from build123d import *

# Parameters (mm, degrees)
SHELL1_OUTLINE_R        = 79.375
SHELL1_DEPTH            = 31.75
CUT_EXTRUDE2_REACH      = 143.848
CUT_EXTRUDE2_END_RADIUS = 92.075


# Read off the part's stored shape, not the designer's step: Shell1
with BuildPart() as part:
    # Sketch1 → Revolve1 (revolve)
    with BuildSketch(Plane.XY, mode=Mode.PRIVATE) as revolve1_sk:
        Polygon((0, 0), (92.075, 0), (92.075, 19.05), (95.25, 19.05), (95.25, 44.45), (0, 44.45), align=None)
    revolve(revolve1_sk.sketch.rotate(Axis((0, 0, 0), (0, 1, 0)), 90), axis=Axis((0, 0, 0), (0, 1, 0)))

    # Shell1 outline → Shell1 (cut)
    with BuildSketch(Plane(origin=(0, 0, 0), x_dir=(1, 0, 0), z_dir=(0, 1, 0))):
        Circle(SHELL1_OUTLINE_R)
    extrude(amount=SHELL1_DEPTH, mode=Mode.SUBTRACT)

    # Cut-Extrude2: up to this cylinder (the profile starts inside it)
    cut_extrude2_end = Plane(origin=(0, 0, 0), z_dir=(0, -1, 0)) * Cylinder(CUT_EXTRUDE2_END_RADIUS, 472.846, mode=Mode.PRIVATE)
    # Sketch2 → Cut-Extrude2 (cut, up to the surface)
    with BuildSketch(Plane(origin=(0, 0, 0), x_dir=(0, 0, -1), z_dir=(1, 0, 0)), mode=Mode.PRIVATE) as cut_extrude2_sk1:
        with BuildLine():
            Line((-48.830201285, -11.43), (-48.830201285, 11.43))
            ThreePointArc((-48.830201285, 11.43), (-42.480201285, 17.78), (-36.130201285, 11.43))
            Line((-36.130201285, 11.43), (-36.130201285, -11.43))
            ThreePointArc((-36.130201285, -11.43), (-42.480201285, -17.78), (-48.830201285, -11.43))
        make_face()
    cut_extrude2_tool1 = extrude(cut_extrude2_sk1.sketch, amount=CUT_EXTRUDE2_REACH, mode=Mode.PRIVATE) & cut_extrude2_end
    add(cut_extrude2_tool1.solids().sort_by_distance((0, 0, 42.480201))[0], mode=Mode.SUBTRACT)
    # Sketch2 → Cut-Extrude2 (cut, up to the surface)
    with BuildSketch(Plane(origin=(0, 0, 0), x_dir=(0, 0, -1), z_dir=(1, 0, 0)), mode=Mode.PRIVATE) as cut_extrude2_sk2:
        with BuildLine():
            Line((15.101598715, -11.43), (15.101598715, 11.43))
            ThreePointArc((15.101598715, 11.43), (21.451598715, 17.78), (27.801598715, 11.43))
            Line((27.801598715, 11.43), (27.801598715, -11.43))
            ThreePointArc((27.801598715, -11.43), (21.451598715, -17.78), (15.101598715, -11.43))
        make_face()
    cut_extrude2_tool2 = extrude(cut_extrude2_sk2.sketch, amount=CUT_EXTRUDE2_REACH, mode=Mode.PRIVATE) & cut_extrude2_end
    add(cut_extrude2_tool2.solids().sort_by_distance((0, 0, -21.451599))[0], mode=Mode.SUBTRACT)


solid = part.part
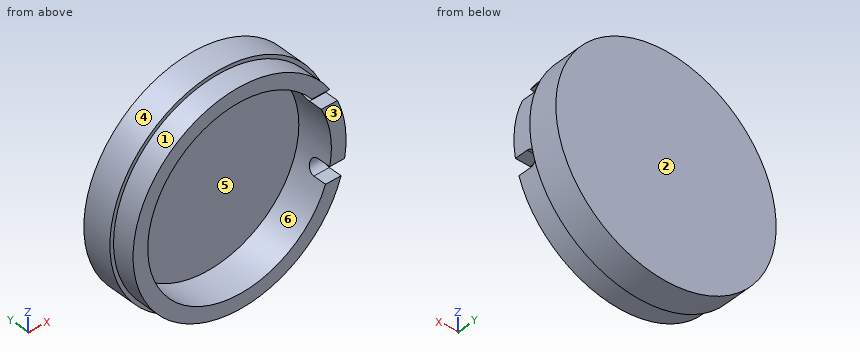
Can you work these out from the model? Positions are in its coordinate system, mm. Face numbers are marked on the shaded views. A direction names the side the tool comes from. Round coordinates to 2 decimals unless told otherwise and drop trailing zeros. Write each loop counter-clockwise with the first axis right and the second up, starting at its lowest first coordinate (ties: lowest second). Pieces come first, ordered by that corner, then holes. Notation, with made-up numbers: (-24, -15.75) -> (4, -15.75) arc R9 ccw to (4, -8.75) -> close; hole circle Ø9 at (40, 32.5). An arc over 180 degrees is marked (long way). Use one line per item in the form item = value. Start each with the question number.
Q1. Imagine slicing it at B-B (z = 0). Please give me the cut outline in (x, y) (3 decimals).
Q2. If I drill on probe 1 along X at (y, z) = (15, 0) (3 decimals); probe 2 along X at (y, z) = (22, 0) (3 decimals); probe 3 along Y at (x, z) = (14, -31.5), over which ranges is the centre line in solid material (lowest first)? Write a range as [from, to].
Q3. We'd pull the mould along Z, two halves only. Please class the marked faces 3, 4, 5 and 6: +Z half, -Z half, draft (parallel to the pull), parting line (faces both ways), or undercut.
Q4. Imagine slicing it at C-C (x = 0). Please give me the cut outline in (y, z) (3 decimals), then the cut area to 3 significant figures.
Q5. I'm going to push flat-ended pins straight in: P1, Ø1.5, axis at x = -27.5, y = 21, coming from the -Z side; P2, Ø3.5, axis at x = 80.5, y = 8.5, coming from the +Z side; P3, Ø1.5, axis at y = 38.5, z = 64, coming from the -X side. Where does each tip first touch, or does it pass through?
Q6. Imagine slicing it at D-D (y = 28). Please give me the cut outline in (x, z) (3 decimals).
Q7. Which directions (+Z, -Z, +X, -X, +Y, -Y) give clear straight access to the entire face, cutting with the end or side of a thin tool? Please do the marked faces 1 and 2.
Q8. Imagine slicing it at A-A (y = 4). Please give me the cut outline in (x, z) (3 decimals).
Worked out:
q1.outline = (-95.25, 19.05) -> (-92.075, 19.05) -> (-92.075, 0) -> (-79.375, 0) -> (-79.375, 31.75) -> (79.375, 31.75) -> (79.375, 0) -> (92.075, 0) -> (92.075, 19.05) -> (95.25, 19.05) -> (95.25, 44.45) -> (-95.25, 44.45) -> close
q2.probe_1 = [-92.075, -79.375], [79.375, 92.075]
q2.probe_2 = [-95.25, -79.375], [79.375, 95.25]
q2.probe_3 = [31.75, 44.45]
q3.face_3 = draft
q3.face_4 = parting line
q3.face_5 = undercut
q3.face_6 = undercut
q4.outline = (0, -92.075) -> (19.05, -92.075) -> (19.05, -95.25) -> (44.45, -95.25) -> (44.45, 95.25) -> (19.05, 95.25) -> (19.05, 92.075) -> (0, 92.075) -> (0, 79.375) -> (31.75, 79.375) -> (31.75, -79.375) -> (0, -79.375) -> close
q4.area = 3,310 mm^2
q5.P1 = -91.42
q5.P2 = 36.13
q5.P3 = -71.22
q6.outline = circle Ø190.5 at (0, 0); hole circle Ø158.75 at (0, 0)
q7.face_1 = -Y
q7.face_2 = +Z, -Z, +X, -X, +Y
q8.outline = (62.578, 48.83) -> (78.06, 48.83) arc R92.075 ccw (long way) to (87.777, -27.802) -> (74.347, -27.802) arc R79.375 cw (long way) to start; (70.675, 36.13) arc R79.375 cw to (77.925, -15.102) -> (90.828, -15.102) arc R92.075 ccw to (84.69, 36.13) -> close
